Study the drawing (mm; zero at the part's minimum x, y, z) and answer. A direction names the side the tool comes from. Coordinates: 2 decimals unless noted, no trailing zeros. Order: outer loops, then holes, each group sorted by start corner. A loop starts at its lowest first (then second) coordinate and runs counter-clockwise, first axis right, second up. Notation, with made-up numbers: M 44.5,20 L 71.5,20 A21 ccw 71.5,31 Z; hole C -17.75,-14 d9. An arc over 180 degrees is marked long. One line per item, written item: value. Start each with the question number.
Q1. The part is cut by section A-A on x = 25.4. Give the vertices of the cut face in (y, z) (3 decimals), then the cut area to 3 significant figures.
Q2. The part is cut by section C-C on y = 11.5. Give the vertices of the cut face in (x, z) (3 decimals), then the cut area to 3 significant figures.
Q3. The part is cut by section B-B on z = 12.5. Give the vertices of the cut face in (x, y).
Q4. For the marked faces 1, 2 and 3, determine the directions among +Z, -Z, +X, -X, +Y, -Y from which every point of the face is accessible in a straight line to the end or side of a thin tool.
Q5. Each of these flat-tipped pins is pushed along its axis until it touches: pin 1 Ø1 at (x, z) = (39, 23.5) entering from -Y; pin 2 Ø10 at (y, z) = (12, 27.5) entering from +X; pin 3 Ø11.5 at (x, y) = (25, 51.5) entering from +Z; pin 4 Ø10 at (x, y) = (25.4, 38.1) entering from +Z. Where does it stop, or does it pass through?
Q6. Determine the mould class of the marked faces 4, 5 and 6 for opening direction X: pulls with the +X half, pulls with the -X half, needs draft (parallel to the pull), parting line crosses it, or undercut.
Q7. The part is cut by section D-D on x = 41. Give the vertices of the cut face in (y, z) (3 decimals).
Q8. Straight lines are drawn through the part: line 1 along Y through (x, z) = (25, 31.5); line 2 along X through (y, z) = (38.1, 29.5); line 3 along Y through (x, z) = (25, 20). For each, find the intervals that lie inside material, in ascending order. Write a range as [from, to].
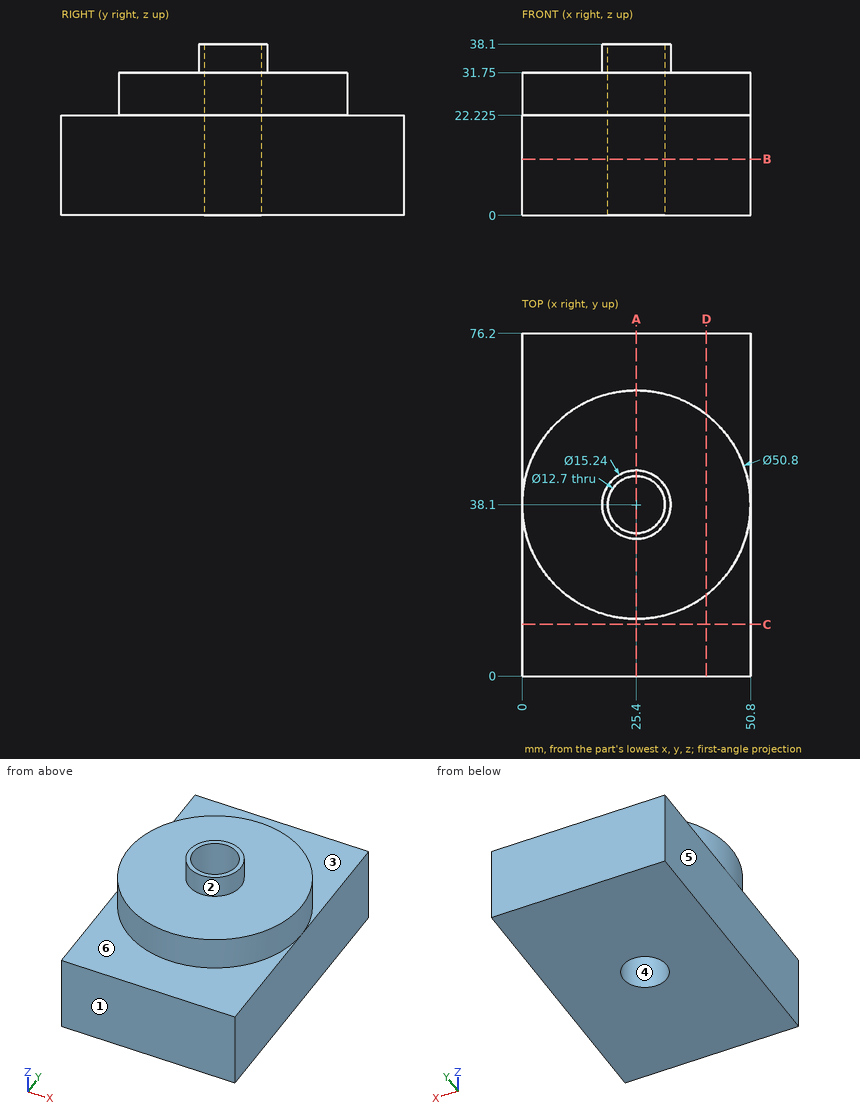
Output:
1. outline: M 0,0 L 31.75,0 L 31.75,38.1 L 30.48,38.1 L 30.48,31.75 L 12.7,31.75 L 12.7,22.225 L 0,22.225 Z; M 44.45,0 L 76.2,0 L 76.2,22.225 L 63.5,22.225 L 63.5,31.75 L 45.72,31.75 L 45.72,38.1 L 44.45,38.1 Z
1. area: 1,790 mm^2
2. outline: M 0,0 L 50.8,0 L 50.8,22.225 L 0,22.225 Z
2. area: 1,130 mm^2
3. outline: M 0,0 L 50.8,0 L 50.8,76.2 L 0,76.2 Z; hole C 25.4,38.1 d12.7
4. face 1: +Z, -Z, +X, -X, -Y
4. face 2: +Z
4. face 3: +Z, +Y
5. pin 1: stops at y = 16.34
5. pin 2: stops at x = 39.54
5. pin 3: stops at z = 31.75
5. pin 4: passes through
6. face 4: undercut
6. face 5: pulls with the -X half
6. face 6: needs draft
7. outline: M 0,0 L 76.2,0 L 76.2,22.225 L 58.145,22.225 L 58.145,31.75 L 18.055,31.75 L 18.055,22.225 L 0,22.225 Z
8. line 1: y = [12.7, 31.76], [44.44, 63.5]
8. line 2: x = [0, 19.05], [31.75, 50.8]
8. line 3: y = [0, 31.76], [44.44, 76.2]
